Model file for the job. Use its own axes, mm. Face numbers are marked on the shaded views. A direction names the side the tool comes from. Round coordinates to 2 decimals unless told otherwise and drop trailing zeros. Write each loop counter-clockwise with the first axis right and the second up, starting at its lowest first coordinate (ties: lowest second). Pieces come first, ordered by that corner, then holes. Notation, with made-up numbers: (-29.75, 70.5) - (10.25, 70.5) arc R17 ccw to (10.25, 87.5) - close; hole circle Ø1 at (13, 30.25). An arc over 180 degrees is marked (long way). Answer as a JSON object with one key per item and string values. Group by question number.
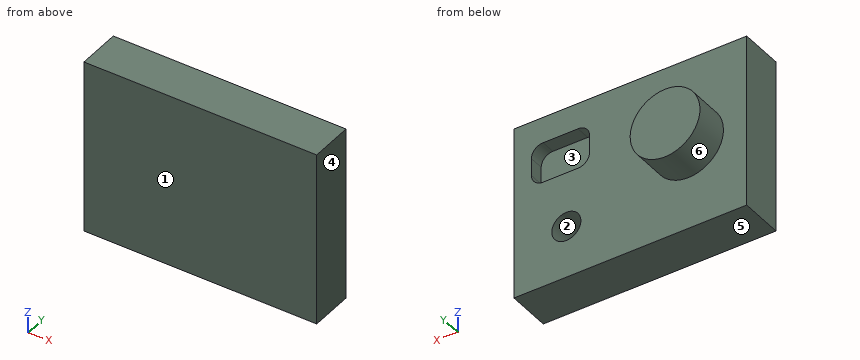
from build123d import *

# Parameters (mm, degrees)
SKETCH1_W           = 80
SKETCH1_H           = 60
BOSS_EXTRUDE1_DEPTH = 15
SKETCH2_R           = 12
BOSS_EXTRUDE2_DEPTH = 12
SKETCH3_R           = 5
CUT_EXTRUDE2_DEPTH  = 10
CUT_EXTRUDE4_DEPTH  = 5


with BuildPart() as part:
    # Sketch1 → Boss-Extrude1 (new body)
    with BuildSketch(Plane(origin=(0, 0, 0), x_dir=(1, 0, 0), z_dir=(0, 1, 0))):
        Rectangle(SKETCH1_W, SKETCH1_H)
    extrude(amount=BOSS_EXTRUDE1_DEPTH)

    # Sketch2 → Boss-Extrude2 (add)
    with BuildSketch(Plane(origin=(0, 15, 0), x_dir=(1, 0, 0), z_dir=(0, 1, 0))):
        with Locations(Location((-20, 0, 0), (0, 0, 270))):
            Circle(SKETCH2_R)
    extrude(amount=BOSS_EXTRUDE2_DEPTH)

    # Sketch3 → Cut-Extrude2 (cut)
    with BuildSketch(Plane(origin=(0, 15, 0), x_dir=(1, 0, 0), z_dir=(0, 1, 0))):
        with Locations(Location((22, 12, 0), (0, 0, 270))):
            Circle(SKETCH3_R)
    extrude(amount=-CUT_EXTRUDE2_DEPTH, mode=Mode.SUBTRACT)

    # Sketch4 → Cut-Extrude4 (cut)
    with BuildSketch(Plane(origin=(0, 15, 0), x_dir=(1, 0, 0), z_dir=(0, 1, 0))):
        with BuildLine():
            Line((18, -21), (30, -21))
            ThreePointArc((30, -21), (32.828427125, -19.828427125), (34, -17))
            Line((34, -17), (34, -11))
            ThreePointArc((34, -11), (32.828427125, -8.171572875), (30, -7))
            Line((30, -7), (18, -7))
            ThreePointArc((18, -7), (15.171572875, -8.171572875), (14, -11))
            Line((14, -11), (14, -17))
            ThreePointArc((14, -17), (15.171572875, -19.828427125), (18, -21))
        make_face()
    extrude(amount=-CUT_EXTRUDE4_DEPTH, mode=Mode.SUBTRACT)


solid = part.part
(1) Slice it at C-C (z = 0). Write the cut outline in (x, y), then the cut area to 3 significant figures.
(2) Drill centre lines: line 1 (X direction, y = 9, z = -12); line 2 (Y direction, x = 24.5, z = -5.5); line 3 (Z direction, x = 18.5, y = 12.25). Where is each one in solid material? Low to high. Write a range as from..to.
(3) Flat gauge pins, fed straight in: pin 1 (6 mm diameter, centred on x = 22, z = -12, fed in from +Y); pin 2 (4 mm diameter, centred on x = 7, z = -18.5, fed in from -Y); pin 3 (7 mm diameter, centred on x = 22.5, z = 16, fed in from +Y); pin 4 (8 mm diameter, centred on x = -16, z = 23, fed in from +Y). Where does each tip first touch, or does it go through?
(4) 3-axis set-ups, long thin cutter, end or side, ignore diameter. For the marked faces 5 and 6: which of +Z, -Z, +X, -X, +Y, -Y reach the whole face in a straight line?
(5) Slice it at D-D (y = 6.25). Write the cut outline in (x, z), then the cut area to 3 significant figures.
(6) Slice it at B-B (x = 22). Write the cut outline in (y, z).
(7) Pull direction X, two halves, no side cores. Call the marked faces 1, 2, 3 and 4: pulls with the +X half, pulls with the -X half, needs draft (parallel to the pull), parting line crosses it, or undercut.
(8) Slice it at A-A (y = 12.5). Write the cut outline in (x, z).
Answer:
{
 "1": {"outline": "(-40, 0) - (40, 0) - (40, 15) - (-8, 15) - (-8, 27) - (-32, 27) - (-32, 15) - (-40, 15) - close", "area": "1,490 mm²"},
 "2": {"line 1": "-40..17, 27..40", "line 2": "0..15", "line 3": "-30..-15.57, -8.43..7, 21..30"},
 "3": {"pin 1": "y = 5", "pin 2": "y = 0", "pin 3": "y = 10", "pin 4": "y = 15"},
 "4": {"face 5": "-Z, +X, -X, +Y, -Y", "face 6": "+Y"},
 "5": {"outline": "(-40, -30) - (40, -30) - (40, 30) - (-40, 30) - close; hole circle Ø10 at (22, -12)", "area": "4,720 mm²"},
 "6": {"outline": "(0, -30) - (15, -30) - (15, -17) - (5, -17) - (5, -7) - (15, -7) - (15, 7) - (10, 7) - (10, 21) - (15, 21) - (15, 30) - (0, 30) - close"},
 "7": {"face 1": "needs draft", "face 2": "undercut", "face 3": "undercut", "face 4": "pulls with the +X half"},
 "8": {"outline": "(-40, -30) - (40, -30) - (40, 30) - (-40, 30) - close; hole (14, 11) arc R4 ccw to (18, 7) - (30, 7) arc R4 ccw to (34, 11) - (34, 17) arc R4 ccw to (30, 21) - (18, 21) arc R4 ccw to (14, 17) - close; hole circle Ø10 at (22, -12)"}
}
